Could you check a few things on this model? Use its own coordinates, in mm. Face numbers are marked on the shaded views. A direction names the side the tool comes from. Round coordinates to 2 decimals unless told otherwise and drop trailing zeros. Order: outer loops, then holes, each group sorted by start corner. A loop starts at its lowest first (then second) coordinate and runs counter-clockwise, first axis right, second up. Notation, with made-up numbers: (47, -26) - (60, -26) arc R34 ccw to (60, 12) - close; hole circle Ø1 at (31, -11). An arc over 180 degrees is marked (long way). Use one line per item in the form item = value.
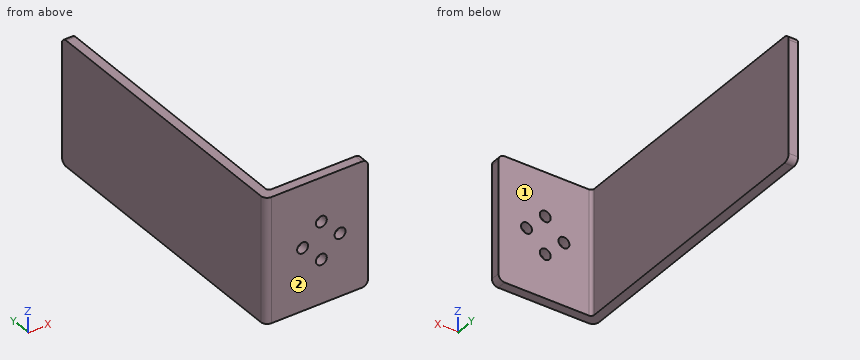
from build123d import *

# Parameters (mm, degrees)
EXTRU_MINCE1_DEPTH      = 40
CONG_1_R                = 1
CONG_2_R                = 2
CONG_3_R                = 2
CONG_4_R                = 2
CONG_5_R                = 2
CONG_6_R                = 2
ESQUISSE3_R             = 1.75
ENL_V_MAT_EXTRU_2_DEPTH = 10


with BuildPart() as part:
    # Esquisse1 → Extru.-Mince1 (new body)
    with BuildSketch(Plane.XY):
        Polygon((30, 0), (0, 0), (0, 90), (-3, 90), (-3, -3), (30, -3), align=None)
    extrude(amount=EXTRU_MINCE1_DEPTH)

    # Congé1
    cong_1_edges = [part.edges().sort_by_distance(p)[0] for p in [
        (0, 0, 20),
    ]]
    fillet(cong_1_edges, radius=CONG_1_R)

    # Congé2
    cong_2_edges = [part.edges().sort_by_distance(p)[0] for p in [
        (-3, -3, 20),
    ]]
    fillet(cong_2_edges, radius=CONG_2_R)

    # Congé3
    cong_3_edges = [part.edges().sort_by_distance(p)[0] for p in [
        (-1.5, 90, 40),
    ]]
    fillet(cong_3_edges, radius=CONG_3_R)

    # Congé4
    cong_4_edges = [part.edges().sort_by_distance(p)[0] for p in [
        (-1.5, 90, 0),
    ]]
    fillet(cong_4_edges, radius=CONG_4_R)

    # Congé5
    cong_5_edges = [part.edges().sort_by_distance(p)[0] for p in [
        (30, -1.5, 40),
    ]]
    fillet(cong_5_edges, radius=CONG_5_R)

    # Congé6
    cong_6_edges = [part.edges().sort_by_distance(p)[0] for p in [
        (30, -1.5, 0),
    ]]
    fillet(cong_6_edges, radius=CONG_6_R)

    # Esquisse3 → Enlèv. mat.-Extru.2 (cut)
    with BuildSketch(Plane(origin=(0, 0, 0), x_dir=(1, 0, 0), z_dir=(0, 1, 0))):
        with Locations(Location((15, -14, 0), (0, 0, 270))):
            Circle(ESQUISSE3_R)
        with Locations(Location((15, -26, 0), (0, 0, 270))):
            Circle(ESQUISSE3_R)
        with Locations(Location((21, -20, 0), (0, 0, 270))):
            Circle(ESQUISSE3_R)
        with Locations(Location((9, -20, 0), (0, 0, 270))):
            Circle(ESQUISSE3_R)
    extrude(amount=-ENL_V_MAT_EXTRU_2_DEPTH, mode=Mode.SUBTRACT)


solid = part.part
Item 1: Will these pins go through, and if not, where does the flat tip stop? P1, Ø4, axis at x = 15, z = 26, coming from the +Y side; P2, Ø6, axis at x = 1.5, y = 25, coming from the -Z side; P3, Ø3, axis at x = 21, z = 20, coming from the +Y side; P4, Ø1, axis at y = 53.5, z = 17, coming from the +X side.
Found:
P1 = 0
P2 = 0
P3 = through
P4 = 0
Item 2: Imagine slicing it at B-B on z = 26. Please give me the cut outline in (x, y).
Found:
outline = (-3, -1) arc R2 ccw to (-1, -3) - (13.25, -3) - (13.25, 0) - (1, 0) arc R1 cw to (0, 1) - (0, 90) - (-3, 90) - close; (16.75, -3) - (30, -3) - (30, 0) - (16.75, 0) - close
Item 3: For the marked faces 1 and 2, which set-ups out of +Z, -Z, +X, -X, +Y, -Y let a thin tool reach every point of the face, with its end or its side?
Found:
face_1 = +Z, -Z, +X, +Y
face_2 = +Z, -Z, +X, -X, -Y
Item 4: Imagine slicing it at D-D on z = 20. Please give me the cut outline in (x, y).
Found:
outline = (-3, -1) arc R2 ccw to (-1, -3) - (7.25, -3) - (7.25, 0) - (1, 0) arc R1 cw to (0, 1) - (0, 90) - (-3, 90) - close; (10.75, -3) - (19.25, -3) - (19.25, 0) - (10.75, 0) - close; (22.75, -3) - (30, -3) - (30, 0) - (22.75, 0) - close
Item 5: Imagine slicing it at A-A on x = 15. Please give me the cut outline in (y, z), plus the area to 3 significant figures.
Found:
outline = (-3, 0) - (0, 0) - (0, 12.25) - (-3, 12.25) - close; (-3, 15.75) - (0, 15.75) - (0, 24.25) - (-3, 24.25) - close; (-3, 27.75) - (0, 27.75) - (0, 40) - (-3, 40) - close
area = 99.0 mm2
Item 6: Imagine slicing it at C-C on x = 21. Please give me the cut outline in (y, z), plus the area to 4 significant figures.
Found:
outline = (-3, 0) - (0, 0) - (0, 18.25) - (-3, 18.25) - close; (-3, 21.75) - (0, 21.75) - (0, 40) - (-3, 40) - close
area = 109.5 mm2
Item 7: I need wall thicknesses on L1, parallel to X at y = -0.8, z = 14; L2, parallel to Y at x = 2.5, z = 29.5. Which ranges of each line are inside material? Lowest first, please.
Found:
L1 = -3 to 13.25, 16.75 to 30
L2 = -3 to 0
